The listing builds one solid part. Answer for the finished solid, in the listing's coordinates (mm). Face numbers are marked on the shaded views. A direction names the side the tool comes from. Give positions to 0.01 mm unless a question says otherwise; leave off trailing zeros. Write each loop counter-clockwise with the first axis right and the second up, starting at its lowest first coordinate (ties: lowest second). Pieces come first, ordered by that corner, then holes. Notation, with made-up numbers: (-35, 19) - (-11, 19) arc R14 cw to (-11, 43) - close; hole circle Ø4 at (9.25, -30.75). An arc over 180 degrees is marked (long way). One line per question, with ' | ' between items. Start each with the question number.
1. Find the intervals of material crossed by L1, parallel to X at y = 27.5, z = 23; L2, parallel to X at y = 75.5, z = 44.5; L3, parallel to Z at x = -215, y = 249.5, in increasing order. Write a range as from..to.
2. A cutting plane is placed at A-A (y = 73). Determine the outline of the cut face in (x, z).
3. For the marked faces 1, 2 and 3, determine the directions among +Z, -Z, +X, -X, +Y, -Y from which every point of the face is accessible in a straight line to the end or side of a thin tool.
4. The mould has two halves that part along Y. Classify the marked faces 4, 5 and 6: +Y half, -Y half, draft (parallel to the pull), parting line (faces both ways), or undercut.
5. Given P1, Ø10.5, axis at x = -152, y = 271.47, coming from the -Z side; P2, Ø7.5, axis at y = 94.5, z = 69.5, coming from the +X side; P3, Ø10, axis at x = -125.5, z = 57.5, coming from the -Y side; P4, Ø3, axis at x = -117, z = 18.5, coming from the +Y side, each flat-ended and moving along its own axis, determine where each tip first touches the part or whether it passes through.
6. A cutting plane is placed at B-B (z = 60.5). Determine the outline of the cut face in (x, y), then the cut area to 3 significant figures.
7. A cutting plane is placed at D-D (y = 135.5). Determine the outline of the cut face in (x, z), then the cut area to 3 significant figures.
8. A cutting plane is placed at C-C (z = 12.5). Determine the outline of the cut face in (x, y), then the cut area to 3 significant figures.
```python
from build123d import *

# Parameters (mm, degrees)
F0_R     = 6.5405
F1_DEPTH = 76.2
F3_DEPTH = 25.4


with BuildPart() as f1:
    # F0 (on Top) → F1 (new body)
    with BuildSketch(Plane.XY):
        Polygon((-67.9690890407, 110.6476840292), (0, 76.2), (0, 203.2), (-153.9793167929, 292.1), (-274.9630657016, 222.25), (-275.7369360322, 215.9473319371), (-198.2431763687, 176.672411752), (-158.5945410949, 156.5779294016), (-113.2818150678, 133.6128067154), align=None)
        with Locations((-151.9981167929, 271.4667715498)):
            Circle(F0_R, mode=Mode.SUBTRACT)
        with Locations((-20.3835, 196.212271957)):
            Circle(F0_R, mode=Mode.SUBTRACT)
        Polygon((-198.2431763687, 176.672411752), (-275.7369360322, 215.9473319371), (-280.3801580159, 178.1313235595), (-298.267005539, 127.6204243564), (-241.3343504537, 155.5403700614), align=None)
        Polygon((-275.7369360322, 215.9473319371), (-274.9630657016, 222.25), (-300.8671202676, 126.3453202542), (-298.267005539, 127.6204243564), (-280.3801580159, 178.1313235595), align=None)
        Polygon((-189.2178803878, 103.2717895071), (-158.5945410949, 156.5779294016), (-198.2431763687, 176.672411752), (-241.3343504537, 155.5403700614), (-221.8573776706, 46.4561172643), align=None)
        Polygon((-131.5564353, 64.8183334656), (-113.2818150678, 133.6128067154), (-158.5945410949, 156.5779294016), (-189.2178803878, 103.2717895071), (-145.8874004982, 10.8696773813), align=None)
        Polygon((-59.2936250137, -9.6900026026), (-65.6310013179, 78.2159816061), (-67.9690890407, 110.6476840292), (-113.2818150678, 133.6128067154), (-131.5564353, 64.8183334656), align=None)
        Polygon((-65.6310013179, 78.2159816061), (0, 0), (0, 76.2), (-67.9690890407, 110.6476840292), align=None)
    extrude(amount=F1_DEPTH)

    # F2 (on face) → F3 (cut)
    with BuildSketch(Plane.XY.offset(76.2)):
        Polygon((0, 0), (0, 203.2), (-153.9793167929, 292.1), (-274.9630657016, 222.25), (-300.8671202676, 126.3453202542), (-241.3343504537, 155.5403700614), (-221.8573776706, 46.4561172643), (-189.2178803878, 103.2717895071), (-145.8874004982, 10.8696773813), (-131.5564353, 64.8183334656), (-59.2936250137, -9.6900026026), (-65.6310013179, 78.2159816061), align=None)
        with BuildLine():
            Line((-13.8508234279, 196.5320797972), (-12.7, 195.8676515813))
            Line((-12.7, 195.8676515813), (-12.7, 34.8929632271))
            Line((-12.7, 34.8929632271), (-81.1190261519, 116.4315834454))
            Line((-81.1190261519, 116.4315834454), (-74.4697648189, 24.1994303135))
            Line((-74.4697648189, 24.1994303135), (-138.067730519, 89.7736666719))
            Line((-138.067730519, 89.7736666719), (-149.2034024598, 47.8536335482))
            Line((-149.2034024598, 47.8536335482), (-188.0773837652, 130.7522764553))
            Line((-188.0773837652, 130.7522764553), (-215.4882373861, 83.0381201455))
            Line((-215.4882373861, 83.0381201455), (-231.7944080284, 174.363731179))
            Line((-231.7944080284, 174.363731179), (-281.2995293986, 150.0862704018))
            Line((-281.2995293986, 150.0862704018), (-264.0702576195, 213.874268841))
            Line((-264.0702576195, 213.874268841), (-156.9828667929, 275.7012027616))
            ThreePointArc((-156.9828667929, 275.7012027616), (-150.2699352174, 277.774824236), (-145.5512194367, 272.5693388853))
            Line((-145.5512194367, 272.5693388853), (-23.3728765721, 202.0296397432))
            ThreePointArc((-23.3728765721, 202.0296397432), (-17.11325, 201.8765111104), (-13.8508234279, 196.5320797972))
        make_face(mode=Mode.SUBTRACT)
    extrude(amount=-F3_DEPTH, mode=Mode.SUBTRACT)


solid = f1.part
```
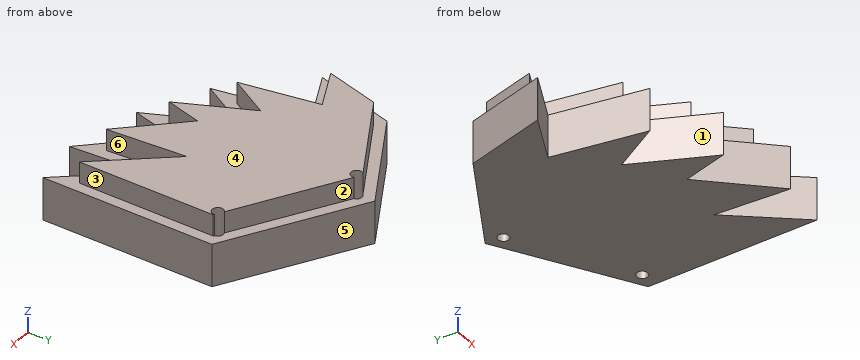
Determined:
1) L1: -153.69..-141.47, -95.36..-61.97, -23.08..0 | L2: -227.04..-205.17, -176.19..-65.44, -63.35..0 | L3: 0..50.8
2) outline: (-226.6, 0) - (-206.61, 0) - (-206.61, 50.8) - (-226.6, 50.8) - close; (-175.02, 0) - (-65.25, 0) - (-65.25, 50.8) - (-77.99, 50.8) - (-77.99, 76.2) - (-121.8, 76.2) - (-121.8, 50.8) - (-142.52, 50.8) - (-142.52, 76.2) - (-161, 76.2) - (-161, 50.8) - (-175.02, 50.8) - close; (-61.25, 0) - (0, 0) - (0, 50.8) - (-12.7, 50.8) - (-12.7, 76.2) - (-44.68, 76.2) - (-44.68, 50.8) - (-61.25, 50.8) - close
3) face 1: +Z, -Z, -Y | face 2: +Z, +X, +Y | face 3: +Z, +X, +Y, -Y
4) face 4: draft | face 5: +Y half | face 6: undercut
5) P1: through | P2: x = -12.7 | P3: y = 71.66 | P4: y = 271.62
6) outline: (-281.3, 150.09) - (-231.79, 174.36) - (-215.49, 83.04) - (-188.08, 130.75) - (-149.2, 47.85) - (-138.07, 89.77) - (-74.47, 24.2) - (-81.12, 116.43) - (-12.7, 34.89) - (-12.7, 195.87) - (-13.85, 196.53) arc R6.54 cw (long way) to (-23.37, 202.03) - (-145.55, 272.57) arc R6.54 cw (long way) to (-156.98, 275.7) - (-264.07, 213.87) - close | area: 37,800 mm2
7) outline: (-298.39, 0) - (-282.2, 0) - (-282.2, 50.8) - (-298.39, 50.8) - close; (-237.76, 0) - (0, 0) - (0, 50.8) - (-12.7, 50.8) - (-12.7, 76.2) - (-224.86, 76.2) - (-224.86, 50.8) - (-237.76, 50.8) - close | area: 18,300 mm2
8) outline: (-300.87, 126.35) - (-241.33, 155.54) - (-221.86, 46.46) - (-189.22, 103.27) - (-145.89, 10.87) - (-131.56, 64.82) - (-59.29, -9.69) - (-65.63, 78.22) - (0, 0) - (0, 203.2) - (-153.98, 292.1) - (-274.96, 222.25) - close; hole circle Ø13.08 at (-152, 271.47); hole circle Ø13.08 at (-20.38, 196.21) | area: 53,300 mm2
